Read the model definition and answer for the solid it produces. Units are mm, in the model's axes. Give positions to 0.01 mm unless a question says otherwise; leave off trailing zeros. Write each loop counter-clockwise with the first axis right and the second up, starting at its lowest first coordinate (ties: lowest second). Pieces come first, ordered by that corner, then holes. Notation, with made-up numbers: (63.25, 44) -> (67.25, 44) arc R14 ccw to (67.25, 56) -> close; hole circle Ø1 at (17.5, 82). An arc over 180 degrees is marked (long way). Put each result on its own line as item: value. Start each with the question number.
from build123d import *

# Parameters (mm, degrees)
DODANIE_WYCI_GNI_CIE1_DEPTH = 0.75


with BuildPart() as part:
    # Szkic2 → Dodanie-wyciągnięcie1 (new body)
    with BuildSketch(Plane.XY):
        with BuildLine():
            Line((-198.180056235, -174.343371382), (-198.180056235, 174.343371382))
            add(Edge.make_bspline(
                [(-198.180056235, 174.343371382), (-198.814001088, 174.406171049), (-200.029378534, 174.610462196), (-202.057107029, 175.259966245), (-203.861424394, 176.203690636), (-205.297190597, 177.249011775), (-206.016868944, 177.898350742), (-206.350638573, 178.234256298)],
                knots=[0.983916118, 0.983916118, 0.983916118, 0.983916118, 1.01810112, 1.052286122, 1.086471125, 1.103563626, 1.120656127, 1.120656127, 1.120656127, 1.120656127], degree=3))
            add(Edge.make_bspline(
                [(-206.350638573, 178.234256298), (-206.752993703, 178.198264306), (-207.539928278, 178.138556667), (-209.26679718, 178.051541981), (-211.615353293, 178.018552884), (-214.778879334, 178.117030022), (-219.442272991, 178.45896865), (-226.083190988, 179.327493296), (-235.041515621, 181.174554614), (-244.401007092, 183.815912629), (-251.88971958, 186.553469872), (-257.317102506, 188.930286392), (-261.034871731, 190.768565716), (-263.783209225, 192.309993434), (-265.771886977, 193.543556647), (-266.665075006, 194.137485785), (-267.11637499, 194.44902024)],
                knots=[0.004638779, 0.004638779, 0.004638779, 0.004638779, 0.015597592, 0.026556404, 0.04847403, 0.070391656, 0.092309282, 0.136144533, 0.179979785, 0.223815036, 0.267650288, 0.289567914, 0.311485539, 0.333403165, 0.344361978, 0.355320791, 0.355320791, 0.355320791, 0.355320791], degree=3))
            Line((-267.11637499, 194.44902024), (-905.657427312, 289.90714954))
            add(Edge.make_bspline(
                [(-905.657427312, 289.90714954), (-906.006104535, 289.315247268), (-906.804551959, 288.159312543), (-908.572469256, 286.249166576), (-911.015586006, 284.522093086), (-913.404414633, 283.603556478), (-915.194323394, 283.225046758), (-916.005259178, 283.136981023), (-916.423901621, 283.11129086)],
                knots=[0.312267878, 0.312267878, 0.312267878, 0.312267878, 0.332062336, 0.351856793, 0.391445708, 0.431034623, 0.450829081, 0.470623538, 0.470623538, 0.470623538, 0.470623538], degree=3))
            Line((-916.423901621, 283.11129086), (-916.423901621, -283.11129086))
            add(Edge.make_bspline(
                [(-916.423901621, -283.11129086), (-916.005259178, -283.136981023), (-915.194323394, -283.225046758), (-913.404414633, -283.603556478), (-911.015586006, -284.522093086), (-908.572469256, -286.249166576), (-906.804551959, -288.159312543), (-906.006104535, -289.315247268), (-905.657427312, -289.90714954)],
                knots=[0.029376462, 0.029376462, 0.029376462, 0.029376462, 0.049170919, 0.068965377, 0.108554292, 0.148143207, 0.167937664, 0.187732122, 0.187732122, 0.187732122, 0.187732122], degree=3))
            Line((-905.657427312, -289.90714954), (-267.11637499, -194.44902024))
            add(Edge.make_bspline(
                [(-267.11637499, -194.44902024), (-266.665075006, -194.137485784), (-265.771886977, -193.543556647), (-263.783209225, -192.309993434), (-261.034871731, -190.768565716), (-257.317102506, -188.930286392), (-251.88971958, -186.553469872), (-244.401007092, -183.815912629), (-235.041515621, -181.174554614), (-226.083190988, -179.327493296), (-219.442272991, -178.45896865), (-214.778879334, -178.117030022), (-211.615353293, -178.018552884), (-209.26679718, -178.051541981), (-207.539928278, -178.138556667), (-206.752993703, -178.198264306), (-206.350638573, -178.234256298)],
                knots=[0.644679209, 0.644679209, 0.644679209, 0.644679209, 0.655638022, 0.666596835, 0.688514461, 0.710432086, 0.732349712, 0.776184964, 0.820020215, 0.863855467, 0.907690718, 0.929608344, 0.95152597, 0.973443596, 0.984402408, 0.995361221, 0.995361221, 0.995361221, 0.995361221], degree=3))
            add(Edge.make_bspline(
                [(-206.350638573, -178.234256298), (-206.016868944, -177.898350742), (-205.297190597, -177.249011775), (-203.861424394, -176.203690636), (-202.057107029, -175.259966245), (-200.029378534, -174.610462196), (-198.814001088, -174.406171049), (-198.180056235, -174.343371382)],
                knots=[0.379343873, 0.379343873, 0.379343873, 0.379343873, 0.396436374, 0.413528875, 0.447713878, 0.48189888, 0.516083882, 0.516083882, 0.516083882, 0.516083882], degree=3))
        make_face()
    extrude(amount=DODANIE_WYCI_GNI_CIE1_DEPTH)


solid = part.part
1) A cutting plane is placed at A-A on x = -479. Give the vertices of the cut face in (y, z), and give its area (3 significant figures).
2) Straight lines are drawn through the part: line 1 (Y direction, x = -465.5, z = 0.6); line 2 (X direction, y = -175.5, z = 0.2); line 3 (Y direction, x = -542, z = 0.25). For each, find the intervals that lie inside material, in ascending order. Write a range as [from, to].
3) A cutting plane is placed at B-B on x = -669. Give the vertices of the cut face in (y, z), and give its area (3 significant figures).
Results found:
1. outline: (-226.12, 0) -> (226.12, 0) -> (226.12, 0.75) -> (-226.12, 0.75) -> close
1. area: 339 mm²
2. line 1: y = [-224.11, 224.11]
2. line 2: x = [-916.42, -202.44]
2. line 3: y = [-235.54, 235.54]
3. outline: (-254.53, 0) -> (254.53, 0) -> (254.53, 0.75) -> (-254.53, 0.75) -> close
3. area: 382 mm²
